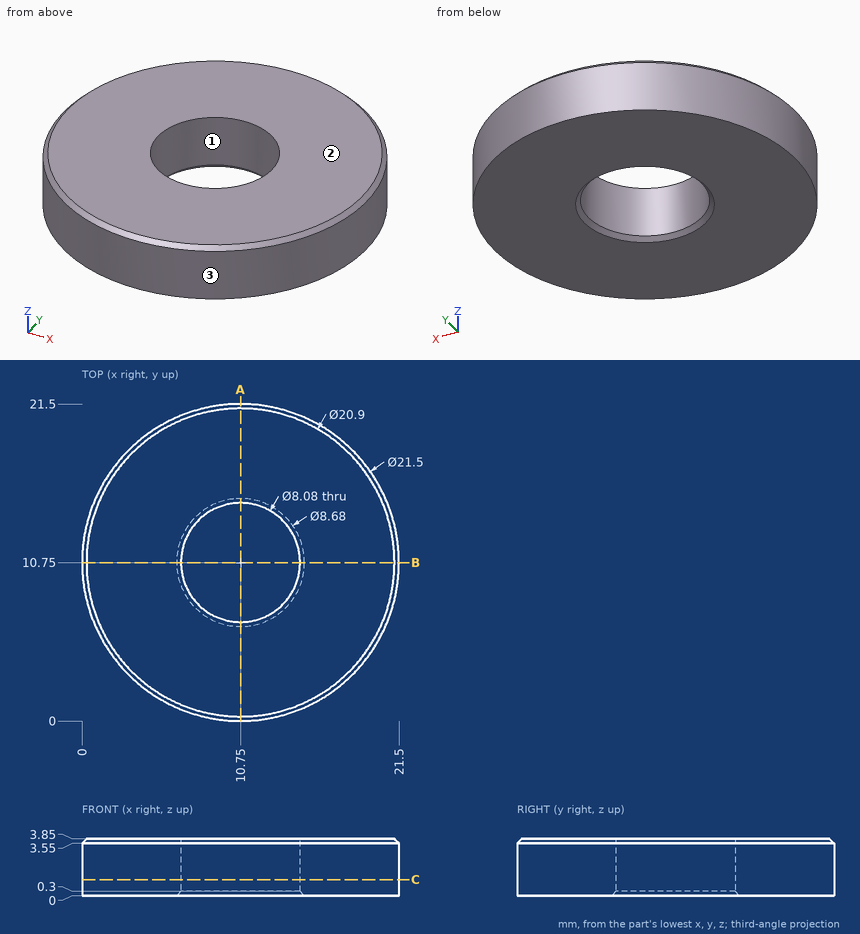
Geometry check sheet. Reference: drawing and pictorial views, mm from the part's lowest x, y, z. Coordinates: 2 decimals unless noted, no trailing zeros. Loops run counter-clockwise (first coordinate to the right, second up) from the corner with the lowest first, then second, coordinate; pieces in that order, holes last.
1) Sectioned sample at A-A (x = 10.75). Record the boundary of the cut face in (y, z), and give its area (3 significant figures).
2) Material ranges on probe 1 along Y at (x, z) = (10.75, 1.8); probe 2 along X at (y, z) = (12.25, 3.5); probe 3 along Y at (x, z) = (8.25, 2.95), recorded low to high.
3) Gauge pin test, flat ends, axial feed: pin 1 (1.5 mm diameter, centred on x = 3, z = 2.5, fed in from -Y); pin 2 (5 mm diameter, centred on x = 10.75, y = 10.75, fed in from +Z). Record the tip position at first contact, or that the pin passes through.
4) Sectioned sample at C-C (z = 1.1). Record the boundary of the cut face in (x, y).
5) Release check for a two-part mould opening along Y. For the marked faces 1, 2 and 3 record: released by +Y, released by -Y, zero draft, split by the parting line, or undercut.
Check sheet entries:
1. outline: (0, 0) - (6.41, 0) - (6.71, 0.3) - (6.71, 3.85) - (0.3, 3.85) - (0, 3.55) - close; (14.79, 0.3) - (15.09, 0) - (21.5, 0) - (21.5, 3.55) - (21.2, 3.85) - (14.79, 3.85) - close
1. area: 51.5 mm2
2. probe 1: y = 0 to 6.71, 14.79 to 21.5
2. probe 2: x = 0.11 to 7, 14.5 to 21.39
2. probe 3: y = 0.29 to 7.58, 13.92 to 21.21
3. pin 1: stops at y = 2.59
3. pin 2: passes through
4. outline: circle Ø21.5 at (10.75, 10.75); hole circle Ø8.08 at (10.75, 10.75)
5. face 1: undercut
5. face 2: zero draft
5. face 3: split by the parting line
